Could you check a few things on this model? Use its own coordinates, in mm. Face numbers are marked on the shaded views. A direction names the side the tool comes from. Coordinates: 2 decimals unless noted, no trailing zeros. Loops run counter-clockwise (first coordinate to the right, second up) from the corner with the lowest first, then second, coordinate; pieces in that order, holes last. Notation, with made-up numbers: (24, 46.5) -> (49, 46.5) arc R21 cw to (49, 67.5) -> close; hole circle Ø11 at (79.25, 64.5). An arc over 180 degrees is marked (long way). One line per question, with ' | ' between items.
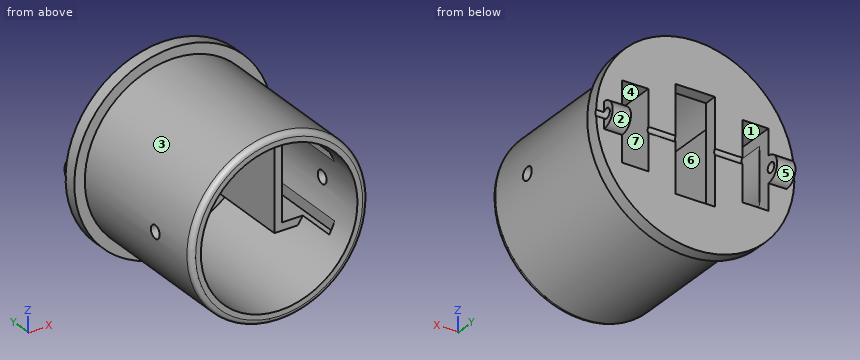
from build123d import *

# Parameters (mm, degrees)
SKETCH1_R               = 43.18
SKETCH1_R_2             = 38.1
BOSS_EXTRUDE1_DEPTH     = 76.2
SKETCH4_R               = 48.26
BOSS_EXTRUDE2_DEPTH     = 6.35
SKETCH5_W               = 19.05
SKETCH5_H               = 50.8
CUT_EXTRUDE2_DEPTH      = 6.35
BOSS_EXTRUDE3_DEPTH     = 8.89
CUT_EXTRUDE3_START      = -12.7
SKETCH7_R               = 2.38125
CUT_EXTRUDE3_DEPTH      = 99.06
CUT_EXTRUDE4_DEPTH      = 48.26
CUT_EXTRUDE4_DEPTH_BACK = 48.26
SKETCH8_R               = 3.175
FILLET2_R               = 2.54
SKETCH11_W              = 12.7
SKETCH11_H              = 38.1
CUT_EXTRUDE5_DEPTH      = 69.85
BOSS_EXTRUDE4_DEPTH     = 44.45


with BuildPart() as part:
    # Sketch1 → Boss-Extrude1 (new body)
    with BuildSketch(Plane(origin=(0, 0, 0), x_dir=(1, 0, 0), z_dir=(0, 1, 0))):
        with Locations(Location((0, 0, 0), (0, 0, 90))):
            Circle(SKETCH1_R)
        with Locations(Location((0, 0, 0), (0, 0, 90))):
            Circle(SKETCH1_R_2, mode=Mode.SUBTRACT)
    extrude(amount=BOSS_EXTRUDE1_DEPTH)

    # Sketch4 → Boss-Extrude2 (add)
    with BuildSketch(Plane(origin=(0, 76.2, 0), x_dir=(1, 0, 0), z_dir=(0, 1, 0))):
        with Locations(Location((0, 0, 0), (0, 0, 270))):
            Circle(SKETCH4_R)
    extrude(amount=BOSS_EXTRUDE2_DEPTH)

    # Sketch5 → Cut-Extrude2 (cut)
    with BuildSketch(Plane(origin=(0, 82.55, 0), x_dir=(1, 0, 0), z_dir=(0, 1, 0))):
        Rectangle(SKETCH5_W, SKETCH5_H)
    extrude(amount=-CUT_EXTRUDE2_DEPTH, mode=Mode.SUBTRACT)

    # Sketch6 → Boss-Extrude3 (add)
    with BuildSketch(Plane(origin=(35.56, 0, 0), x_dir=(0, 0, -1), z_dir=(1, 0, 0))):
        with BuildLine():
            Line((-6.35, 82.55), (6.35, 82.55))
            ThreePointArc((6.35, 82.55), (0, 88.9), (-6.35, 82.55))
        make_face()
    boss_extrude3 = extrude(amount=BOSS_EXTRUDE3_DEPTH)

    # Sketch7 → Cut-Extrude3 (cut)
    with BuildSketch(Plane.ZY.offset(-35.56).offset(CUT_EXTRUDE3_START)):
        with Locations(Location((0, 84.455, 0), (0, 0, 233.130102354))):
            Circle(SKETCH7_R)
    cut_extrude3 = extrude(amount=CUT_EXTRUDE3_DEPTH, mode=Mode.SUBTRACT)

    # Mirror1: Boss-Extrude3, Cut-Extrude3 across plane
    add(boss_extrude3.mirror(Plane(origin=(0, 0, 0), x_dir=(0, 0, 1), z_dir=(1, 0, 0))))
    add(cut_extrude3.mirror(Plane(origin=(0, 0, 0), x_dir=(0, 0, 1), z_dir=(1, 0, 0))), mode=Mode.SUBTRACT)

    # Sketch8 → Cut-Extrude4 (cut, two sides: drawn at the far end of the back side and taken through both)
    with BuildSketch(Plane(origin=(0, 0, 0), x_dir=(0, 0, -1), z_dir=(1, 0, 0)).offset(-CUT_EXTRUDE4_DEPTH_BACK)):
        with Locations(Location((0, 25.4, 0), (0, 0, 180))):
            Circle(SKETCH8_R)
    extrude(amount=CUT_EXTRUDE4_DEPTH + CUT_EXTRUDE4_DEPTH_BACK, mode=Mode.SUBTRACT)

    # Fillet2
    fillet2_edges = [part.edges().sort_by_distance(p)[0] for p in [
        (0, 0, 43.18),
    ]]
    fillet(fillet2_edges, radius=FILLET2_R)

    # Sketch11 → Cut-Extrude5 (cut)
    with BuildSketch(Plane(origin=(0, 82.55, 0), x_dir=(1, 0, 0), z_dir=(0, 1, 0))):
        with Locations((29.21, 0.11160914)):
            Rectangle(SKETCH11_W, SKETCH11_H)
        with Locations((-29.21, 0.11160914)):
            Rectangle(SKETCH11_W, SKETCH11_H)
    extrude(amount=-CUT_EXTRUDE5_DEPTH, mode=Mode.SUBTRACT)

    # Sketch12 → Boss-Extrude4 (add)
    with BuildSketch(Plane.XZ.offset(-76.2)):
        Polygon((-19.05, 22.74839086), (-31.75, 22.74839086), (-33.059754259, 18.93839086), (-22.86, 18.93839086), (-22.86, -19.16160914), (-32.930878141, -19.16160914), (-31.75, -22.97160914), (-19.05, -22.97160914), align=None)
        Polygon((22.86, 18.93839086), (22.86, -19.16160914), (32.930878141, -19.16160914), (31.75, -22.97160914), (19.05, -22.97160914), (19.05, 22.74839086), (31.75, 22.74839086), (33.059754259, 18.93839086), align=None)
    extrude(amount=BOSS_EXTRUDE4_DEPTH)


solid = part.part
1) If we section it at C-C on y = 62.5: Please give me the cut outline in (x, z).
Data:
outline: circle Ø86.36 at (0, 0); hole (-35.56, -19.16) -> (-22.86, -19.16) -> (-22.86, 18.94) -> (-35.56, 18.94) -> (-35.56, 13.68) arc R38.1 ccw to (-35.56, -13.68) -> close; hole (-30.56, 22.75) -> (-19.05, 22.75) -> (-19.05, -22.97) -> (-30.4, -22.97) arc R38.1 ccw to (30.4, -22.97) -> (19.05, -22.97) -> (19.05, 22.75) -> (30.56, 22.75) arc R38.1 ccw to start; hole (22.86, -19.16) -> (35.56, -19.16) -> (35.56, -13.68) arc R38.1 ccw to (35.56, 13.68) -> (35.56, 18.94) -> (22.86, 18.94) -> close
2) I need wall thicknesses on line 1 along X through (y, z) = (76.5, -1) (3 decimals); line 2 along X through (y, z) = (71, 0); line 3 along Z through (x, y) = (27.5, 64). Which ranges of each line are inside material? Lowest first, please. Write a range as from..to.
Data:
line 1: -48.25..-35.56, -22.86..-9.525, 9.525..22.86, 35.56..48.25 | line 2: -43.18..-38.1, -22.86..-19.05, 19.05..22.86, 38.1..43.18 | line 3: -33.29..-26.37, -22.97..-19.16, 18.94..22.75, 26.37..33.29
3) If we section it at B-B on x = 0: Please give me the cut outline in (y, z), and give its area (3 significant figures).
Data:
outline: (0, -40.64) arc R2.54 ccw to (2.54, -43.18) -> (76.2, -43.18) -> (76.2, -48.26) -> (82.55, -48.26) -> (82.55, -25.4) -> (76.2, -25.4) -> (76.2, -38.1) -> (0, -38.1) -> close; (0, 38.1) -> (76.2, 38.1) -> (76.2, 25.4) -> (82.55, 25.4) -> (82.55, 48.26) -> (76.2, 48.26) -> (76.2, 43.18) -> (2.54, 43.18) arc R2.54 ccw to (0, 40.64) -> close | area: 1,060 mm²
4) If we section it at A-A on y = 16: Please give me the cut outline in (x, z).
Data:
outline: circle Ø86.36 at (0, 0); hole (-35.56, -19.16) -> (-32.93, -19.16) arc R38.1 ccw to (32.93, -19.16) -> (35.56, -19.16) -> (35.56, -13.68) arc R38.1 ccw to (35.56, 13.68) -> (35.56, 18.94) -> (33.06, 18.94) arc R38.1 ccw to (-33.06, 18.94) -> (-35.56, 18.94) -> (-35.56, 13.68) arc R38.1 ccw to (-35.56, -13.68) -> close
5) If we section it at D-D on z = 0: Give the number of separate pieces and of enclosed holes in the cut face, and give its area (3 significant figures).
Data:
separate pieces: 8 | enclosed holes: 0 | area: 1,390 mm²
6) I'm going to push flat-ended pins straight in: pin 1 Ø10 at (x, y) = (-29, 60.5) entering from -Z; pin 2 Ø5 at (x, y) = (-16.5, 49) entering from +Z; pin 3 Ø13.5 at (y, z) = (64.5, 2) entering from +X; pin 4 Ø5 at (x, z) = (-35.5, 37) entering from -Y. Where does each tip first touch, or does it pass through?
Data:
pin 1: z = -35.9 | pin 2: z = 40.85 | pin 3: x = 43.18 | pin 4: through
7) We'd pull the mould along X, two halves only. Please class the marked faces 1, 2 and 3: pulls with the +X half, pulls with the -X half, needs draft (parallel to the pull), parting line crosses it, or undercut.
Data:
face 1: undercut | face 2: needs draft | face 3: parting line crosses it
8) On a 3-axis mill with a long thin cutter (end or side, diameter ignored), from which of +Z, -Z, +X, -X, +Y, -Y can I reach the whole of each face in a straight line? I mean the marked faces 4, 5, 6 and 7. Say none if no direction works.
Data:
face 4: +Y | face 5: +X, -X, +Y | face 6: -Y | face 7: +Y, -Y
